Drawing for the job (mm, zero at the part's lowest x, y, z). A direction names the side the tool comes from. Give positions to 0.01 mm unless a question says otherwise; leave off trailing zeros. Write each loop counter-clockwise with the first axis right and the second up, starting at its lowest first coordinate (ties: lowest second). Pieces come first, ordered by that corner, then holes. Notation, with made-up numbers: (-30.5, -13.75) - (12.5, -13.75) arc R23 ccw to (12.5, 8.25) - close; hole circle Ø1 at (17, 73.5). An arc over 180 degrees is marked (long way). Use CSV: the item, a comma, the result in double quotes.
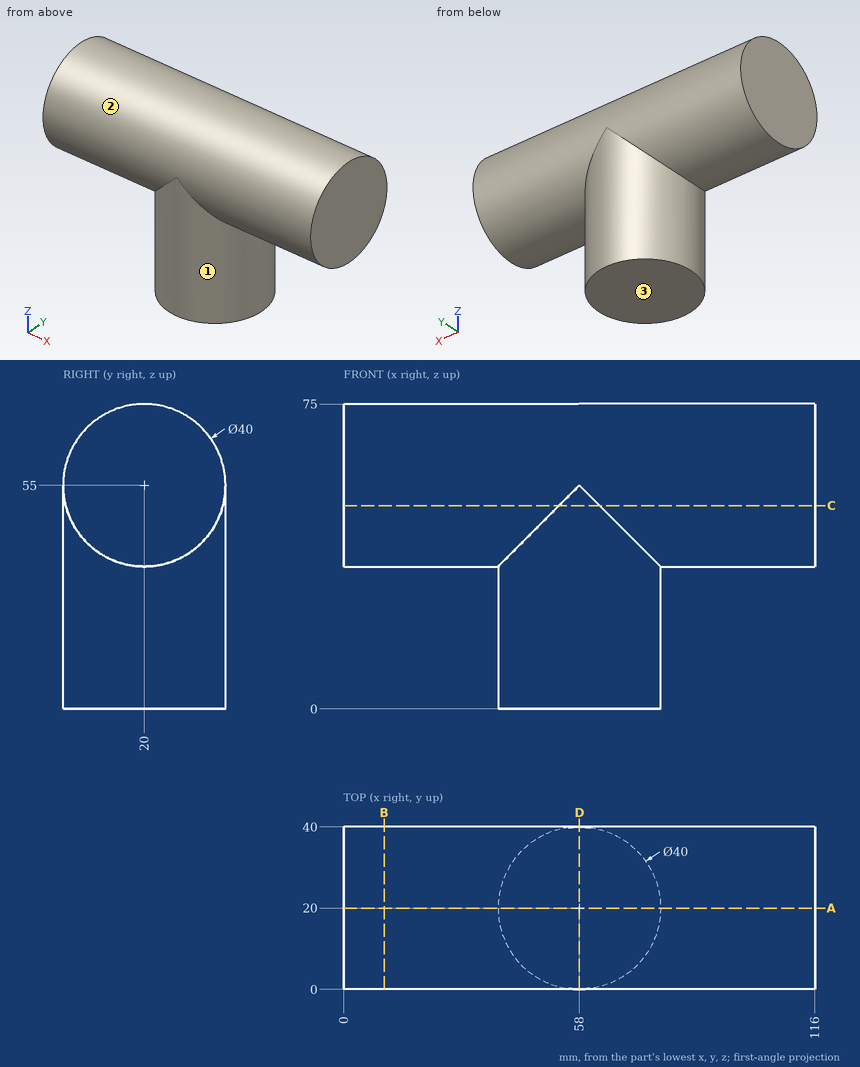
(1) Saw through at A-A, the plane y = 20. List the corners of the cut face in (x, z).
Checked values:
outline,"(0, 35) - (38, 35) - (38, 0) - (78, 0) - (78, 35) - (116, 35) - (116, 75) - (0, 75) - close"
(2) Flat gauge pins, fed straight in: P1, Ø1, axis at x = 16.5, y = 7.5, coming from the +Z side; P2, Ø6, axis at x = 78, y = 21.5, coming from the -Z side; P3, Ø12, axis at x = 45, z = 21, coming from the -Y side (3 decimals); P4, Ø10, axis at x = 94.5, y = 35, coming from the +Z side. Where does each tip first touch, or does it go through?
Checked values:
P1,"stops at z = 71"
P2,"stops at z = 0"
P3,"stops at y = 1.265"
P4,"stops at z = 72.32"
(3) 3-axis set-ups, long thin cutter, end or side, ignore diameter. For the marked faces 1, 2 and 3: which of +Z, -Z, +X, -X, +Y, -Y reach the whole face in a straight line?
Checked values:
face 1,"-Z"
face 2,"none"
face 3,"-Z, +X, -X, +Y, -Y"
(4) Saw through at C-C, the plane z = 50. List the corners of the cut face in (x, y), then the cut area to 3 significant figures.
Checked values:
outline,"(0, 0.64) - (53, 0.64) arc R20 ccw to (63, 0.64) - (116, 0.64) - (116, 39.36) - (63, 39.36) arc R20 ccw to (53, 39.36) - (0, 39.36) - close"
area,"4,500 mm^2"
(5) Saw through at B-B, the plane x = 10. List the corners of the cut face in (y, z).
Checked values:
outline,"circle Ø40 at (20, 55)"
(6) Wall check: probe 1 along Y at (x, z) = (41, 54); probe 2 along Z at (x, y) = (56, 16); probe 3 along Z at (x, y) = (65.5, 27) (3 decimals). Give the ranges that are in metal, low to high. Write a range as [from, to].
Checked values:
probe 1,"y = [0.03, 39.97]"
probe 2,"z = [0, 74.6]"
probe 3,"z = [0, 73.735]"
(7) Saw through at D-D, the plane x = 58. List the corners of the cut face in (y, z).
Checked values:
outline,"(0, 0) - (40, 0) - (40, 55) arc R20 ccw to (0, 55) - close"
